Answer from the drawing. Dimensions are ordinates in mm from the lowest x, y and z of the part. Coordinates: 2 decimals unless noted, no trailing zeros. Loops run counter-clockwise (first coordinate to the right, second up) from the corner with the lowest first, then second, coordinate; pieces in that order, holes last.
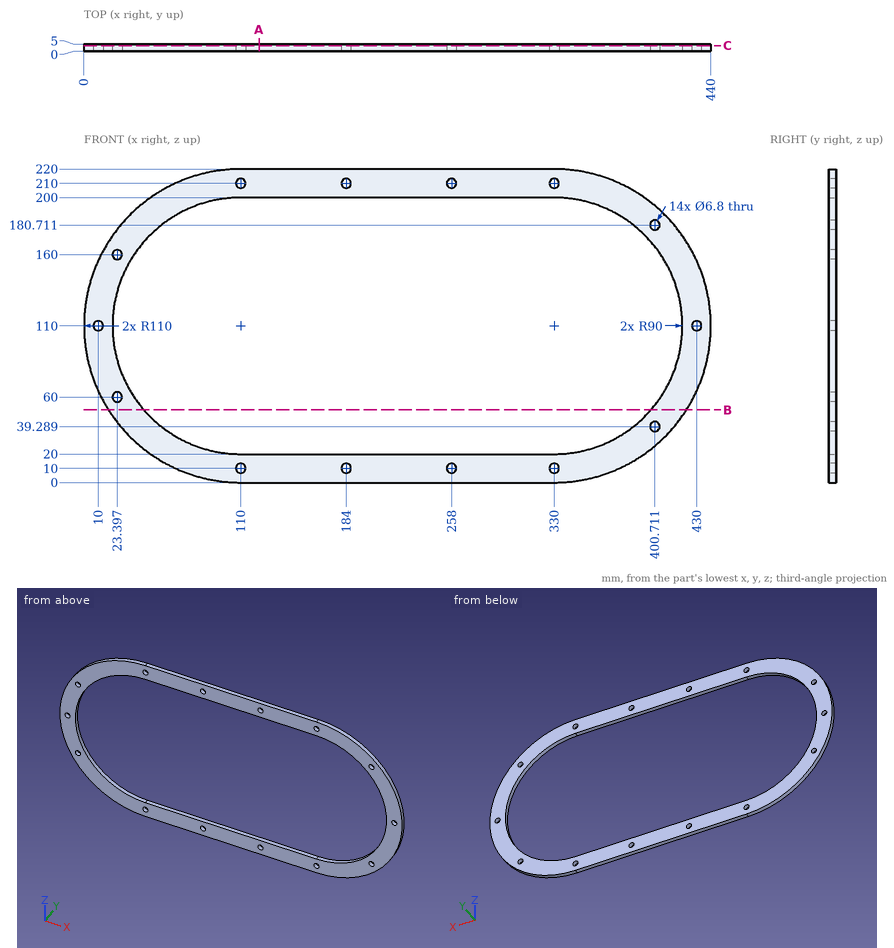
Item 1: A cutting plane is placed at A-A on x = 123. Determine the outline of the cut face in (y, z), then the cut area to 3 significant figures.
Numbers:
outline: (0, 0) - (5, 0) - (5, 20) - (0, 20) - close; (0, 200) - (5, 200) - (5, 220) - (0, 220) - close
area: 200 mm2
Item 2: Find the intervals of material crossed by line 1 along Z through (x, y) = (330, 3.9); line 2 along Z through (x, y) = (297.5, 3.95); line 3 along X through (y, z) = (3.8, 210) (1 decimal), in increasing order.
Numbers:
line 1: z = 0 to 6.6, 13.4 to 20, 200 to 206.6, 213.4 to 220
line 2: z = 0 to 20, 200 to 220
line 3: x = 64.2 to 106.6, 113.4 to 180.6, 187.4 to 254.6, 261.4 to 326.6, 333.4 to 375.8
Item 3: Given pin 1 (1 mm diameter, centred on y = 2, z = 167, fed in from +X), flat-ended and moving along its own axis, determine where the tip first touches the part or whether it passes through.
Numbers:
pin 1: stops at x = 424.38
Item 4: A cutting plane is placed at C-C on y = 3.85. Give the number of separate pieces and of enclosed holes in the cut face, then the cut area to 3 significant figures.
Numbers:
separate pieces: 1
enclosed holes: 15
area: 20,900 mm2
Item 5: A cutting plane is placed at B-B on z = 51. Determine the outline of the cut face in (x, y).
Numbers:
outline: (17.16, 0) - (42.04, 0) - (42.04, 5) - (17.16, 5) - close; (397.96, 0) - (422.84, 0) - (422.84, 5) - (397.96, 5) - close
